Check sheet for the modelled part. Datum: model origin and axes. Units: mm. A direction names the side the tool comes from. Round coordinates to 2 decimals unless told otherwise and drop trailing zeros. Write each loop counter-clockwise with the first axis right and the second up, starting at its lowest first coordinate (ties: lowest second). Pieces come first, ordered by that corner, then holes. Notation, with made-up numbers: (-27.75, -14) - (-2.75, -14) arc R17 cw to (-2.75, 1) - close; hole circle Ø2 at (68.5, 64.25). An arc over 180 degrees is marked (long way). Use one line per item in the form item = value. Start each with the question number.
1) Set-up check for faces 1 (the face through (-0.066, 41.007, -12.907)), 2 (the face through (0, 69, -29.289)), 3 (the face through (12.192, 68, -22.7)): record each of +Z, -Z, +X, -X, +Y, -Y from which the full face is reachable in a straight line by a thin tool's end or side.
2) Section check B-B (x = 0). Record the boundary of the cut face in (y, z) (3 decimals), then the cut area to 3 significant figures.
3) Draft check along Z on faces 4 (the face through (-0.171, 66.884, -25.426)), 5 (the face through (-12.192, 68, -22.7)), 6 (the face through (0.178, 93.56, -28.536)). Enter one of: +Z half, -Z half, draft (parallel to the pull), parting line (faces both ways), or undercut.
4) Scan lines: probe 1 along X at (y, z) = (21, -9.5); probe 2 along X at (y, z) = (80.5, -17); probe 3 along Z at (x, y) = (0, 81). Record each from-to range of solid material in increasing order.
5) Section check A-A (y = 79.5). Record the boundary of the cut face in (x, z).
6) Section check D-D (y = -35.5). Record the boundary of the cut face in (x, z), then the cut area to 3 significant figures.
7) Section check C-C (y = 22.5). Record the boundary of the cut face in (x, z), then the cut area to 3 significant figures.
8) Gauge pin test, flat ends, axial feed: P1, Ø1, axis at x = 0.5, y = -48, coming from the -Z side; P2, Ø5, axis at y = 68, z = -26.5, coming from the +X side; P3, Ø4, axis at x = -7.5, y = 48, coming from the -Z side. Record the tip position at first contact, or that the pin passes through.
from build123d import *

# Parameters (mm, degrees)
F1_DEPTH       = 12.7
F1_DEPTH_BACK  = 12.7
F2_SIZE        = 5.08
F3_R           = 10.16
F4_DEPTH       = 29.21
F5_R           = 4.7169653767
F6_DEPTH       = 14.478
F7_W           = 6.4129335806
F7_H           = 15.100935474
F8_DEPTH       = 15.494
F8_DEPTH_BACK  = 15.494
F9_R           = 1.905
F10_DEPTH      = 39.878
F11_W          = 6.0101076961
F11_H          = 16.6161805391
F12_DEPTH      = 12.192
F12_DEPTH_BACK = 12.192
F13_R          = 1.9082928371
F14_DEPTH      = 25.4


with BuildPart() as f1:
    # F0 (on Right) → F1 (new body, two sides)
    with BuildSketch(Plane.YZ) as f1_sk:
        with BuildLine():
            Line((102.2577819586, 13.1989740504), (-100.9422180414, -24.5563495133))
            Line((-100.9422180414, -24.5563495133), (-26.1237075026, -27.7993018095))
            ThreePointArc((-26.1237075026, -27.7993018095), (-5.1643274907, -15.6669524817), (14.1464179811, -30.2814870284))
            Line((14.1464179811, -30.2814870284), (51.7638866865, -30.9321125706))
            ThreePointArc((51.7638866865, -30.9321125706), (67.8129634232, -18.702842322), (85.1018259738, -29.1058777742))
            Line((85.1018259738, -29.1058777742), (102.2577819586, -27.9500877853))
            Line((102.2577819586, -27.9500877853), (102.2577819586, 13.1989740504))
        make_face()
    extrude(amount=F1_DEPTH)
    extrude(f1_sk.sketch, amount=-F1_DEPTH_BACK)

    # F2
    f2_edges = [f1.edges().sort_by_distance(p)[0] for p in [
        (12.7, 0.657782, -5.678688),
        (-12.7, 0.657782, -5.678688),
    ]]
    chamfer(f2_edges, length=F2_SIZE)

    # F3 (on face) → F4 (cut)
    with BuildSketch(Plane(origin=(0, 102.2577819586, 0), x_dir=(-1, 0, 0), z_dir=(0, 1, 0))):
        with Locations((0, -10.2422883113)):
            Circle(F3_R)
    extrude(amount=-F4_DEPTH, mode=Mode.SUBTRACT)

    # F5 (on face) → F6 (cut)
    with BuildSketch(Plane(origin=(0, 1.041861913, -5.6073242327), x_dir=(1, 0, 0), z_dir=(0, -0.1826772268, 0.9831729404))):
        with Locations((0, 37.893474102)):
            Circle(F5_R)
    extrude(amount=-F6_DEPTH, mode=Mode.SUBTRACT)

    # F7 (on Right) → F8 (join, two sides)
    with BuildSketch(Plane.YZ) as f8_sk:
        with Locations((-3.2064667903, -21.0316376761)):
            Rectangle(F7_W, F7_H)
    extrude(amount=F8_DEPTH)
    extrude(f8_sk.sketch, amount=-F8_DEPTH_BACK)

    # F9 (on face) → F10 (cut)
    with BuildSketch(Plane.YZ.offset(15.494)):
        with Locations((-3.2832995057, -24.805707857)):
            Circle(F9_R)
    extrude(amount=-F10_DEPTH, mode=Mode.SUBTRACT)

    # F11 (on Right) → F12 (join, two sides)
    with BuildSketch(Plane.YZ) as f12_sk:
        with Locations((68.7134154141, -20.981086418)):
            Rectangle(F11_W, F11_H)
    extrude(amount=F12_DEPTH)
    extrude(f12_sk.sketch, amount=-F12_DEPTH_BACK)

    # F13 (on face) → F14 (cut)
    with BuildSketch(Plane(origin=(-12.192, 0, 0), x_dir=(0, -1, 0), z_dir=(-1, 0, 0))):
        with Locations((-68.646594882, -24.6950872242)):
            Circle(F13_R)
    extrude(amount=-F14_DEPTH, mode=Mode.SUBTRACT)


solid = f1.part
Results are:
q1.face_1 = none
q1.face_2 = -Z, +X, -X, +Y
q1.face_3 = -Z, +X
q2.outline = (-100.942, -24.556) - (-26.124, -27.799) arc R21.886 cw to (-6.413, -15.626) - (-6.413, -28.582) - (0, -28.582) - (0, -16.616) arc R21.886 cw to (14.146, -30.281) - (51.764, -30.932) arc R17.962 cw to (65.708, -18.943) - (65.708, -29.289) - (71.718, -29.289) - (71.718, -18.915) arc R17.962 cw to (73.048, -19.187) - (73.048, -0.082) - (102.258, -0.082) - (102.258, 13.199) - (42.935, 2.177) - (45.58, -12.058) - (36.305, -13.781) - (33.66, 0.453) - close; (76.479, -20.402) arc R17.962 cw to (85.102, -29.106) - (102.258, -27.95) - (102.258, -20.402) - close; hole circle Ø3.81 at (-3.283, -24.806); hole circle Ø3.817 at (68.647, -24.695)
q2.area = 3,340 mm²
q3.face_4 = undercut
q3.face_5 = draft
q3.face_6 = -Z half
q4.probe_1 = -12.7 to 12.7
q4.probe_2 = -12.7 to -7.59, 7.59 to 12.7
q4.probe_3 = -23.46 to -20.4, -0.08 to 9.25
q5.outline = (-12.7, -22.21) - (12.7, -22.21) - (12.7, 3.8) - (7.62, 8.97) - (-7.62, 8.97) - (-12.7, 3.8) - close; hole circle Ø20.32 at (0, -10.24)
q6.outline = (-12.7, -27.39) - (12.7, -27.39) - (12.7, -17.56) - (7.62, -12.4) - (-7.62, -12.4) - (-12.7, -17.56) - close
q6.area = 355 mm²
q7.outline = (-12.7, -30.43) - (12.7, -30.43) - (12.7, -6.79) - (7.62, -1.62) - (-7.62, -1.62) - (-12.7, -6.79) - close
q7.area = 705 mm²
q8.P1 = -26.87
q8.P2 = 12.19
q8.P3 = -30.9
